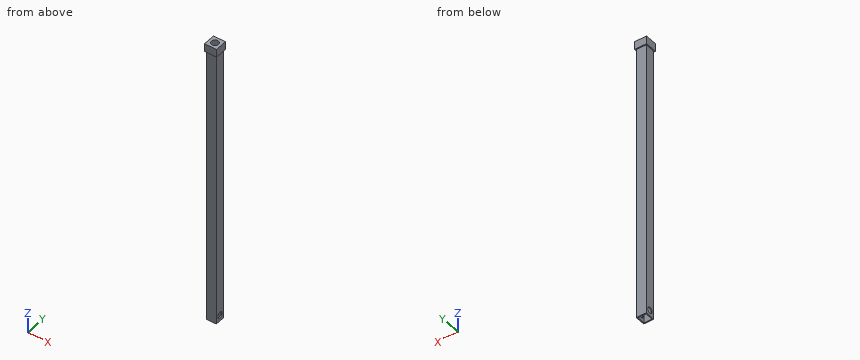
```python
from build123d import *

# Parameters (mm, degrees)
ESQUISSE2_W             = 10
ESQUISSE2_H             = 10
ESQUISSE2_W_2           = 8
ESQUISSE2_H_2           = 8
BOSS_EXTRU_1_DEPTH      = 280
ESQUISSE3_R             = 3
ENL_V_MAT_EXTRU_1_DEPTH = 52
ESQUISSE4_W             = 12
ESQUISSE4_H             = 12
ESQUISSE4_R             = 3.5
BOSS_EXTRU_2_DEPTH      = 8


with BuildPart() as part:
    # Esquisse2 → Boss.-Extru.1 (new body)
    with BuildSketch(Plane.XY):
        Rectangle(ESQUISSE2_W, ESQUISSE2_H)
        Rectangle(ESQUISSE2_W_2, ESQUISSE2_H_2, mode=Mode.SUBTRACT)
    extrude(amount=BOSS_EXTRU_1_DEPTH)

    # Esquisse3 → Enlèv. mat.-Extru.1 (cut)
    with BuildSketch(Plane(origin=(5, 0, 0), x_dir=(0, 0, -1), z_dir=(1, 0, 0))):
        with Locations((-6, 0)):
            Circle(ESQUISSE3_R)
    extrude(amount=-ENL_V_MAT_EXTRU_1_DEPTH, mode=Mode.SUBTRACT)

    # Esquisse4 → Boss.-Extru.2 (add)
    with BuildSketch(Plane.XY.offset(280)):
        Rectangle(ESQUISSE4_W, ESQUISSE4_H)
        Circle(ESQUISSE4_R, mode=Mode.SUBTRACT)
    extrude(amount=BOSS_EXTRU_2_DEPTH)


solid = part.part
```
Design review of the part built by this model. Coordinates are the model's own, in mm. Coordinates: 2 decimals unless noted, no trailing zeros. Order: outer loops, then holes, each group sorted by start corner. A loop starts at its lowest first (then second) coordinate and runs counter-clockwise, first axis right, second up. Notation, with made-up numbers: M -18.75,72.25 L 34.25,72.25 A21 cw 34.25,107.25 Z; hole C 89.5,0.5 d11. An arc over 180 degrees is marked long. Answer as a JSON object with one key per item and string values. Group by question number.
1) Wall thickness on L1, parallel to Y at x = -4.3, z = 6; L2, parallel to Y at x = 1, z = 83: over which ranges is each line inside the solid? List them lowest first.
2) Add section D-D, the plane z = 200.5. Write out the cut boundary in (x, y), then the cut area to 3 significant figures.
3) Add section C-C, the plane y = 0. Write out the cut boundary in (x, z).
4) Add section A-A, the plane z = 6. Write out the cut boundary in (x, y).
5) For pin 1 (5.5 mm diameter, centred on y = 0, z = 6, fed in from -X); pin 2 (3.5 mm diameter, centred on x = 1, y = 1.5, fed in from -Z); pin 3 (7 mm diameter, centred on y = 0, z = 6, fed in from +X); pin 4 (1 mm diameter, centred on x = 3, z = 165, fed in from +Y), all flat-tipped, find the tip position at first contact; note any pin that passes through.
6) Add section B-B, the plane x = 0. Write out the cut boundary in (y, z), then the cut area to 3 significant figures.
Computed values:
{
 "1": {"L1": "y = -5 to -3, 3 to 5", "L2": "y = -5 to -4, 4 to 5"},
 "2": {"outline": "M -5,-5 L 5,-5 L 5,5 L -5,5 Z; hole M -4,-4 L 4,-4 L 4,4 L -4,4 Z", "area": "36.0 mm^2"},
 "3": {"outline": "M -6,280 L -5,280 L -5,9 L -4,9 L -4,280 L -3.5,280 L -3.5,288 L -6,288 Z; M -5,0 L -4,0 L -4,3 L -5,3 Z; M 3.5,280 L 4,280 L 4,9 L 5,9 L 5,280 L 6,280 L 6,288 L 3.5,288 Z; M 4,0 L 5,0 L 5,3 L 4,3 Z"},
 "4": {"outline": "M -5,-5 L 5,-5 L 5,-3 L 4,-3 L 4,-4 L -4,-4 L -4,-3 L -5,-3 Z; M -5,3 L -4,3 L -4,4 L 4,4 L 4,3 L 5,3 L 5,5 L -5,5 Z"},
 "5": {"pin 1": "passes through", "pin 2": "stops at z = 280", "pin 3": "stops at x = 5", "pin 4": "stops at y = 5"},
 "6": {"outline": "M -6,280 L -5,280 L -5,0 L -4,0 L -4,280 L -3.5,280 L -3.5,288 L -6,288 Z; M 3.5,280 L 4,280 L 4,0 L 5,0 L 5,280 L 6,280 L 6,288 L 3.5,288 Z", "area": "600 mm^2"}
}
